Check sheet for the modelled part. Datum: model origin and axes. Units: mm. A direction names the side the tool comes from. Round coordinates to 2 decimals unless told otherwise and drop trailing zeros. Write each loop counter-clockwise with the first axis right and the second up, starting at its lowest first coordinate (ties: lowest second). Pieces come first, ordered by that corner, then holes. Notation, with made-up numbers: (83.25, 2.5) - (101.25, 2.5) arc R6 cw to (101.25, 7.5) - close; hole circle Ø4 at (-19.5, -17). An arc over 180 degrees is marked (long way). Use one line per item in the form item = value. Start each with the question number.
1) Draft check along Z on faces 1 (the face through (84.53, 82.8, -5.72)), 2 (the face through (92.2, 62, 0)), 3 (the face through (86.5, 78, -6)). Enter one of: +Z half, -Z half, draft (parallel to the pull), parting line (faces both ways), or undercut.
2) Scan lines: probe 1 along Y at (x, z) = (83.7, -6); probe 2 along Y at (x, z) = (89.5, -4.5); probe 3 along X at (y, z) = (63.5, -7.5). Record each from-to range of solid material in increasing order.
3) Gauge pin test, flat ends, axial feed: P1, Ø4.5, axis at y = 42.5, z = -6.5, coming from the +X side; P2, Ø2, axis at y = 57, z = -3, coming from the -X side; P3, Ø2, axis at x = 90, z = -1.5, coming from the -Y side. Record the tip position at first contact, or that the pin passes through.
4) Section check D-D (z = -10.25). Record the boundary of the cut face in (x, y), then the cut area to 3 significant figures.
5) Section check B-B (x = 85). Record the boundary of the cut face in (y, z).
6) Section check A-A (z = -6). Record the boundary of the cut face in (x, y), then the cut area to 3 significant figures.
7) Set-up check for faces 4 (the face through (92, 62, -6)), 5 (the face through (86.5, 45, -6)), 6 (the face through (91, 75.668, -6)): record each of +Z, -Z, +X, -X, +Y, -Y from which the full face is reachable in a straight line by a thin tool's end or side.
8) Section check C-C (x = 87.5). Record the boundary of the cut face in (y, z).
from build123d import *

# Parameters (mm, degrees)
BOSS_EXTRUDE1_DEPTH = 12
SKETCH2_R           = 2.15
CUT_EXTRUDE1_DEPTH  = 39


with BuildPart() as part:
    # Sketch1 → Boss-Extrude1 (new body)
    with BuildSketch(Plane.XY):
        Polygon((82.5, 84.667703031), (82.5, 71.767703031), (92, 71.767703031), (92, 51.567703031), (82.5, 51.567703031), (82.5, 38.667703031), (86.5, 38.667703031), (86.5, 47.667703031), (96, 47.667703031), (96, 75.667703031), (86.5, 75.667703031), (86.5, 84.667703031), align=None)
    extrude(amount=-BOSS_EXTRUDE1_DEPTH)

    # Sketch2 → Cut-Extrude1 (cut)
    with BuildSketch(Plane(origin=(86.5, 0, 0), x_dir=(0, 0, -1), z_dir=(1, 0, 0))):
        with Locations((6, 42.667703031)):
            Circle(SKETCH2_R)
        with Locations((6, 80.667703031)):
            Circle(SKETCH2_R)
    extrude(amount=-CUT_EXTRUDE1_DEPTH, mode=Mode.SUBTRACT)


solid = part.part
Results are:
q1.face_1 = undercut
q1.face_2 = +Z half
q1.face_3 = draft
q2.probe_1 = 38.67 to 40.52, 44.82 to 51.57, 71.77 to 78.52, 82.82 to 84.67
q2.probe_2 = 47.67 to 51.57, 71.77 to 75.67
q2.probe_3 = 92 to 96
q3.P1 = 86.5
q3.P2 = 92
q3.P3 = 47.67
q4.outline = (82.5, 38.67) - (86.5, 38.67) - (86.5, 47.67) - (96, 47.67) - (96, 75.67) - (86.5, 75.67) - (86.5, 84.67) - (82.5, 84.67) - (82.5, 71.77) - (92, 71.77) - (92, 51.57) - (82.5, 51.57) - close
q4.area = 258 mm²
q5.outline = (38.67, -12) - (51.57, -12) - (51.57, 0) - (38.67, 0) - close; (71.77, -12) - (84.67, -12) - (84.67, 0) - (71.77, 0) - close; hole circle Ø4.3 at (42.67, -6); hole circle Ø4.3 at (80.67, -6)
q6.outline = (82.5, 38.67) - (86.5, 38.67) - (86.5, 40.52) - (82.5, 40.52) - close; (82.5, 44.82) - (86.5, 44.82) - (86.5, 47.67) - (96, 47.67) - (96, 75.67) - (86.5, 75.67) - (86.5, 78.52) - (82.5, 78.52) - (82.5, 71.77) - (92, 71.77) - (92, 51.57) - (82.5, 51.57) - close; (82.5, 82.82) - (86.5, 82.82) - (86.5, 84.67) - (82.5, 84.67) - close
q6.area = 224 mm²
q7.face_4 = +Z, -Z, -X
q7.face_5 = +Z, -Z, +X, -Y
q7.face_6 = +Z, -Z, +X, +Y
q8.outline = (47.67, -12) - (51.57, -12) - (51.57, 0) - (47.67, 0) - close; (71.77, -12) - (75.67, -12) - (75.67, 0) - (71.77, 0) - close
